```python
from build123d import *

# Parameters (mm, degrees)
ESQUISSE1_W             = 240
ESQUISSE1_H             = 170
BOSS_EXTRU_1_DEPTH      = 5
ESQUISSE2_R             = 1.6
ESQUISSE2_R_2           = 1.5999968
ESQUISSE2_R_3           = 1.607820406
ESQUISSE2_R_4           = 1.25
ENL_V_MAT_EXTRU_1_DEPTH = 5
ESQUISSE3_R             = 1.6
ENL_V_MAT_EXTRU_2_DEPTH = 5
ESQUISSE4_R             = 2.6
ENL_V_MAT_EXTRU_3_DEPTH = 5
ESQUISSE6_W             = 230
ESQUISSE6_H             = 5
BOSS_EXTRU_2_DEPTH      = 40
ESQUISSE8_R             = 10
ENL_V_MAT_EXTRU_4_DEPTH = 5
ESQUISSE9_R             = 10
ENL_V_MAT_EXTRU_5_DEPTH = 10


with BuildPart() as part:
    # Esquisse1 → Boss.-Extru.1 (new body)
    with BuildSketch(Plane.XY):
        with Locations((38.235058845, -76.154688976)):
            Rectangle(ESQUISSE1_W, ESQUISSE1_H)
    extrude(amount=BOSS_EXTRU_1_DEPTH)

    # Esquisse2 → Enlèv. mat.-Extru.1 (cut)
    with BuildSketch(Plane(origin=(0, 0, 0), x_dir=(-1, 0, 0), z_dir=(0, 0, -1))):
        with Locations((-145.2, 4.345311024)):
            Circle(ESQUISSE2_R)
        with Locations((20.538736773, -96.465756273)):
            Circle(ESQUISSE2_R_2)
        with Locations((68.798736773, -90.115756273)):
            Circle(ESQUISSE2_R_2)
        with Locations((69.128665464, -15.430898976)):
            Circle(ESQUISSE2_R_3)
        with Locations((20.632685464, -14.154688976)):
            Circle(ESQUISSE2_R_3)
        with Locations((-31, -87)):
            Circle(ESQUISSE2_R_4)
        with Locations((-11, -87)):
            Circle(ESQUISSE2_R_4)
        with Locations((-31, -13)):
            Circle(ESQUISSE2_R_4)
        with Locations((-11, -13)):
            Circle(ESQUISSE2_R_4)
    extrude(amount=-ENL_V_MAT_EXTRU_1_DEPTH, mode=Mode.SUBTRACT)

    # Esquisse3 → Enlèv. mat.-Extru.2 (cut)
    with BuildSketch(Plane.XY.offset(5)):
        with Locations((57.3, -147.154688976)):
            Circle(ESQUISSE3_R)
    extrude(amount=-ENL_V_MAT_EXTRU_2_DEPTH, mode=Mode.SUBTRACT)

    # Esquisse4 → Enlèv. mat.-Extru.3 (cut)
    with BuildSketch(Plane(origin=(0, 0, 0), x_dir=(-1, 0, 0), z_dir=(0, 0, -1))):
        with Locations((73.764941155, -153.154688976)):
            Circle(ESQUISSE4_R)
        with Locations((-150.235058845, -153.154688976)):
            Circle(ESQUISSE4_R)
        with Locations((-150.235058845, 0.845311024)):
            Circle(ESQUISSE4_R)
        with Locations((73.764941155, 0.845311024)):
            Circle(ESQUISSE4_R)
    extrude(amount=-ENL_V_MAT_EXTRU_3_DEPTH, mode=Mode.SUBTRACT)

    # Esquisse6 → Boss.-Extru.2 (add)
    with BuildSketch(Plane(origin=(0, 0, 0), x_dir=(-1, 0, 0), z_dir=(0, 0, -1))):
        with Locations((-38.235058845, -158.654688976)):
            Rectangle(ESQUISSE6_W, ESQUISSE6_H)
    extrude(amount=BOSS_EXTRU_2_DEPTH)

    # Esquisse8 → Enlèv. mat.-Extru.4 (cut)
    with BuildSketch(Plane.XZ.offset(161.154688976)):
        with Locations(Location((-41.764941155, -20, 0), (0, 0, 270))):
            Circle(ESQUISSE8_R)
        with Locations(Location((-11.764941155, -20, 0), (0, 0, 270))):
            Circle(ESQUISSE8_R)
        with Locations(Location((18.235058845, -20, 0), (0, 0, 270))):
            Circle(ESQUISSE8_R)
    extrude(amount=-ENL_V_MAT_EXTRU_4_DEPTH, mode=Mode.SUBTRACT)

    # Esquisse9 → Enlèv. mat.-Extru.5 (cut)
    with BuildSketch(Plane(origin=(0, 0, 0), x_dir=(-1, 0, 0), z_dir=(0, 0, -1))):
        with Locations((51.764941155, -136.154688976)):
            Circle(ESQUISSE9_R)
        with Locations((21.764941155, -136.154688976)):
            Circle(ESQUISSE9_R)
        with Locations((-8.235058845, -136.154688976)):
            Circle(ESQUISSE9_R)
    extrude(amount=-ENL_V_MAT_EXTRU_5_DEPTH, mode=Mode.SUBTRACT)


solid = part.part
```
The listing builds one solid part. Answer for the finished solid, in the listing's coordinates (mm). A direction names the side the tool comes from. Give positions to 0.01 mm unless a question says otherwise; leave off trailing zeros. Order: outer loops, then holes, each group sorted by start corner. A loop starts at its lowest first (then second) coordinate and runs counter-clockwise, first axis right, second up. Notation, with made-up numbers: (13, -7.5) -> (27, -7.5) arc R30 cw to (27, 17.5) -> close; hole circle Ø8 at (42, -0.5). An arc over 180 degrees is marked (long way). Answer as a JSON object with one key per item and string values. Group by question number.
Item 1: The part is cut by section D-D on z = -7. Write down the section's boundary in (x, y), and give its area (3 significant figures).
Item 2: The part is cut by section B-B on x = -14.5. Write down the section's boundary in (y, z).
Item 3: Determine the mould class of faces 3 (the cylindrical face through (-8.761, -158.69, -29.538)), 4 (the flat face through (40, -156.155, -20)), 5 (the flat face through (-76.765, -159, -20)) for opening direction X: pulls with the +X half, pulls with the -X half, needs draft (parallel to the pull), parting line crosses it, or undercut.
Item 4: A tool of negligible diameter and unlimited length cuts with its end or side. For faces 1 (the flat face through (153.235, -159, -20)), 2 (the flat face through (158.235, -77, 2)), from which of +Z, -Z, +X, -X, +Y, -Y can it reach the whole face along a straight path? Write none if from no direction.
Item 5: Flat-ended cylindrical pins translate along their axes: pin 1 (23 mm diameter, centred on x = -21.76, y = -136.15, fed in from +Z); pin 2 (10 mm diameter, centred on x = 65.5, z = -6.5, fed in from +Y); pin 3 (4 mm diameter, centred on x = 46.5, y = -142.5, fed in from -Z); pin 4 (1.5 mm diameter, centred on y = -160, z = -19, fed in from -X). Find the tip coordinate at first contact, or state that the pin passes through.
Item 6: The part is cut by section C-C on y = -80. Write down the section's boundary in (x, z).
Item 7: The part is cut by section A-A on x = -54.5. Write down the section's boundary in (y, z), and give its area (3 significant figures).
Item 8: Consider L1, parallel to Y at x = 31, z = 3.1; L2, parallel to Y at x = 57.3, z = 1.1; L3, parallel to Z at x = 61, y = -63. Determine where each line is inside the solid, lowest interval first. Write a range as from..to.
Result set:
{
 "1": {"outline": "(-76.76, -161.15) -> (153.24, -161.15) -> (153.24, -156.15) -> (-76.76, -156.15) -> close", "area": "1,150 mm²"},
 "2": {"outline": "(-161.15, -40) -> (-156.15, -40) -> (-156.15, -29.62) -> (-161.15, -29.62) -> close; (-161.15, -10.38) -> (-156.15, -10.38) -> (-156.15, 0) -> (-143.03, 0) -> (-143.03, 5) -> (-161.15, 5) -> close; (-129.28, 0) -> (8.85, 0) -> (8.85, 5) -> (-129.28, 5) -> close"},
 "3": {"face 3": "undercut", "face 4": "needs draft", "face 5": "pulls with the -X half"},
 "4": {"face 1": "-Z, +X, +Y, -Y", "face 2": "+Z, -Z, +X, +Y, -Y"},
 "5": {"pin 1": "z = 5", "pin 2": "y = -156.15", "pin 3": "z = 0", "pin 4": "x = -76.76"},
 "6": {"outline": "(-81.76, 0) -> (158.24, 0) -> (158.24, 5) -> (-81.76, 5) -> close"},
 "7": {"outline": "(-161.15, -40) -> (-156.15, -40) -> (-156.15, 0) -> (-145.77, 0) -> (-145.77, 5) -> (-161.15, 5) -> close; (-126.54, 0) -> (8.85, 0) -> (8.85, 5) -> (-126.54, 5) -> close", "area": "954 mm²"},
 "8": {"L1": "-161.15..-88.25, -85.75..-14.25, -11.75..8.85", "L2": "-161.15..-148.75, -145.55..8.85", "L3": "0..5"}
}
